Build history of the part. All positions in model axes, mm. A direction names the side the tool comes from. Give positions to 0.01 mm unless a question says otherwise; leave off trailing zeros. Write each loop counter-clockwise with the first axis right and the second up, starting at its lowest first coordinate (ties: lowest second). Pieces come first, ordered by that corner, then holes. Notation, with made-up numbers: (-8, 60) -> (28, 60) arc R18 ccw to (28, 72) -> close; hole circle Ø5 at (-23, 10). An arc over 180 degrees is marked (long way). One line per question, with ' | ' between items. Start each with the question number.
(1) Pin check, flat tips, straight feed: P1, Ø5, axis at x = 20, y = 25, coming from the -Z side; P2, Ø22, axis at x = 25.5, z = 22, coming from the -Y side; P3, Ø10, axis at x = 40, y = 16.5, coming from the -Z side; P4, Ø13.5, axis at x = 54, y = 21.5, coming from the +Z side. Stop position of each tip, or through.
(2) Pull direction Y, two halves, no side cores. Call faces 1 (the cylindrical face through (64.054, 26.277, 2.479)), 2 (the cylindrical face through (16.868, 27.872, 2.479)), 3 (the flat face through (39, 0, 2)), 4 (the flat face through (31, 50, 25)): released by +Y, released by -Y, zero draft, split by the parting line, or undercut.
(3) Band-saw the part on C-C, the plane y = 11. Give the cut face in (x, z).
(4) Tool access for faces 5 (the flat face through (0, 36, 3)), 6 (the flat face through (39, 45, 17)): list every direction of +Z, -Z, +X, -X, +Y, -Y with a clear straight run to the whole face (end or side of a thin tool).
(5) Drill centre lines: probe 1 along Y at (x, z) = (60, 3); probe 2 along Z at (x, y) = (40, 48); probe 3 along Y at (x, z) = (18, 27). Where is each one in solid material? Low to high. Write a range as from..to.
(6) Band-saw the part on D-D, the plane z = 16. Give the cut face in (x, y), and give its area (3 significant figures).
(7) Band-saw the part on A-A, the plane y = 25. Give the cut face in (x, z).
(8) Band-saw the part on B-B, the plane x = 40. Give the cut face in (y, z), and give its area (3 significant figures).
from build123d import *

# Parameters (mm, degrees)
F0_W     = 80
F0_H     = 50
F0_R     = 4.25
F1_DEPTH = 5
F2_W     = 80
F2_H     = 5
F3_DEPTH = 45
F4_R     = 8.5
F5_DEPTH = 25
F6_SIZE  = 1
F7_R     = 0.5


with BuildPart() as f1:
    # F0 (on Top) → F1 (new body)
    with BuildSketch(Plane.XY):
        with Locations((40, 25)):
            Rectangle(F0_W, F0_H)
        with Locations((20, 25)):
            Circle(F0_R, mode=Mode.SUBTRACT)
        with Locations((60, 25)):
            Circle(F0_R, mode=Mode.SUBTRACT)
    extrude(amount=F1_DEPTH)

    # F2 (on face) → F3 (join)
    with BuildSketch(Plane.XY.offset(5)):
        with Locations((40, 47.5)):
            Rectangle(F2_W, F2_H)
    extrude(amount=F3_DEPTH)

    # F4 (on face) → F5 (cut)
    with BuildSketch(Plane.XZ.offset(-45)):
        with Locations((40, 28.5)):
            Circle(F4_R)
    extrude(amount=-F5_DEPTH, mode=Mode.SUBTRACT)

    # F6
    f6_edges = [f1.edges().sort_by_distance(p)[0] for p in [
        (31.5, 45, 28.5),
        (31.5, 50, 28.5),
        (15.75, 25, 5),
        (55.75, 25, 5),
        (55.75, 25, 0),
        (15.75, 25, 0),
    ]]
    chamfer(f6_edges, length=F6_SIZE)

    # F7
    f7_edges = [f1.edges().sort_by_distance(p)[0] for p in [
        (40, 50, 50),
        (0, 47.5, 50),
        (40, 45, 50),
        (80, 47.5, 50),
        (0, 50, 25),
        (0, 45, 27.5),
        (0, 22.5, 5),
        (0, 0, 2.5),
        (0, 25, 0),
        (80, 0, 2.5),
        (40, 0, 0),
        (40, 0, 5),
        (80, 22.5, 5),
        (80, 45, 27.5),
        (80, 50, 25),
        (80, 25, 0),
        (40, 50, 0),
    ]]
    fillet(f7_edges, radius=F7_R)


solid = f1.part
Results:
1) P1: passes through | P2: stops at y = 45 | P3: stops at z = 0 | P4: stops at z = 5
2) face 1: undercut | face 2: undercut | face 3: released by -Y | face 4: released by +Y
3) outline: (0, 0.5) arc R0.5 ccw to (0.5, 0) -> (79.5, 0) arc R0.5 ccw to (80, 0.5) -> (80, 4.5) arc R0.5 ccw to (79.5, 5) -> (0.5, 5) arc R0.5 ccw to (0, 4.5) -> close
4) face 5: +Z, -Z, -X, +Y, -Y | face 6: +Z, +X, -X, -Y
5) probe 1: y = 0..20.75, 29.25..50 | probe 2: z = 0..20, 37..50 | probe 3: y = 45..50
6) outline: (0, 45.5) arc R0.5 ccw to (0.5, 45) -> (79.5, 45) arc R0.5 ccw to (80, 45.5) -> (80, 49.5) arc R0.5 ccw to (79.5, 50) -> (0.5, 50) arc R0.5 ccw to (0, 49.5) -> close | area: 400 mm²
7) outline: (0, 0.5) arc R0.5 ccw to (0.5, 0) -> (14.75, 0) -> (15.75, 1) -> (15.75, 4) -> (14.75, 5) -> (0.5, 5) arc R0.5 ccw to (0, 4.5) -> close; (24.25, 1) -> (25.25, 0) -> (54.75, 0) -> (55.75, 1) -> (55.75, 4) -> (54.75, 5) -> (25.25, 5) -> (24.25, 4) -> close; (64.25, 1) -> (65.25, 0) -> (79.5, 0) arc R0.5 ccw to (80, 0.5) -> (80, 4.5) arc R0.5 ccw to (79.5, 5) -> (65.25, 5) -> (64.25, 4) -> close
8) outline: (0, 0.5) arc R0.5 ccw to (0.5, 0) -> (49.5, 0) arc R0.5 ccw to (50, 0.5) -> (50, 19) -> (49, 20) -> (46, 20) -> (45, 19) -> (45, 5) -> (0.5, 5) arc R0.5 ccw to (0, 4.5) -> close; (45, 38) -> (46, 37) -> (49, 37) -> (50, 38) -> (50, 49.5) arc R0.5 ccw to (49.5, 50) -> (45.5, 50) arc R0.5 ccw to (45, 49.5) -> close | area: 388 mm²
